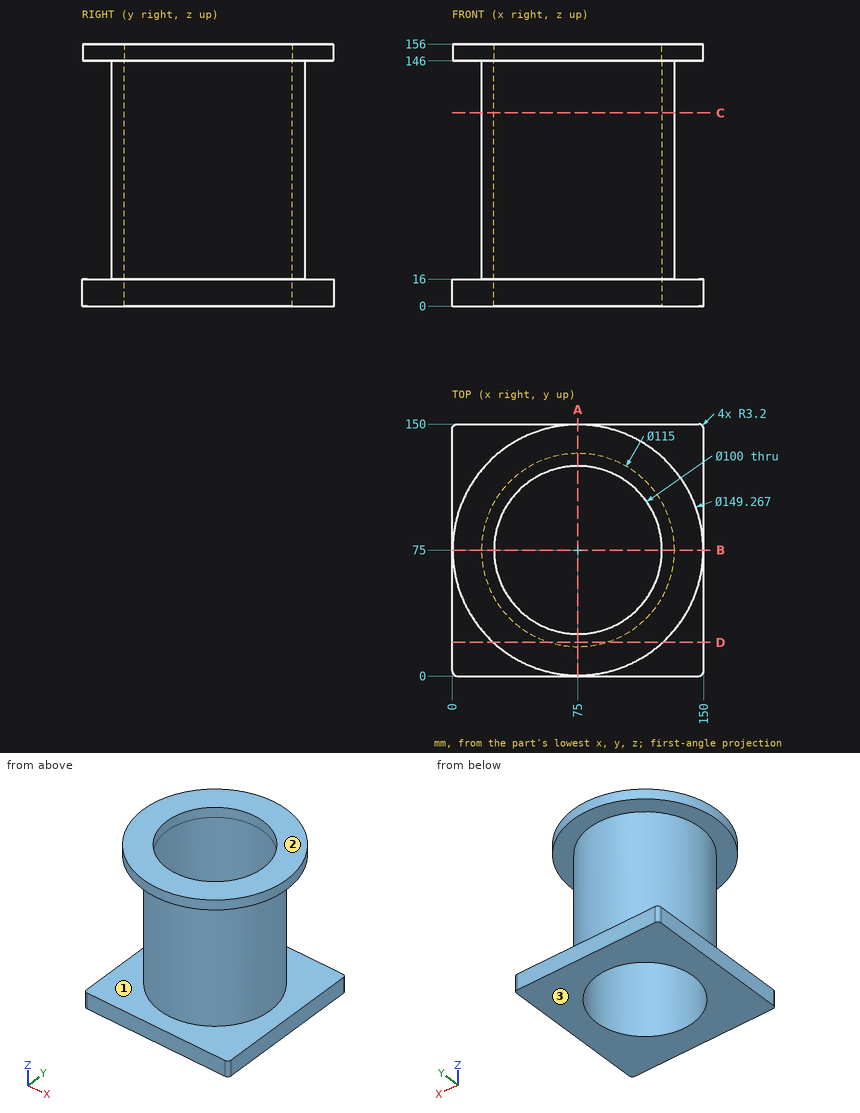
Here's the drawing with two shaded views (mm, measured from the low corner). I have some questions. Give positions to 0.01 mm unless a question says otherwise; leave off trailing zeros. Write each loop counter-clockwise with the first axis right and the second up, starting at its lowest first coordinate (ties: lowest second). Pieces come first, ordered by that corner, then holes. Notation, with made-up numbers: (-11, 16) -> (12, 16) arc R25 ccw to (12, 29) -> close; hole circle Ø4 at (37, -6.75). An arc over 180 degrees is marked (long way). Answer as a JSON object with one key per item and string values. Group by question number.
Item 1: We'd pull the mould along Z, two halves only. Please class the marked faces 1, 2 and 3: +Z half, -Z half, draft (parallel to the pull), parting line (faces both ways), or undercut.
Item 2: I'm going to push flat-ended pins straight in: P1, Ø8, axis at y = 127.5, z = 93.5, coming from the -X side; P2, Ø8, axis at y = 76, z = 34, coming from the -X side; P3, Ø4, axis at y = 89.5, z = 101.5, coming from the -X side (3 decimals). Where does each tip first touch, or does it pass through?
Item 3: Suppose I cut it at C-C (z = 115). Please give me the cut outline in (x, y).
Item 4: Please list where these lines run through material, in increasing order: line 1 (Z direction, x = 105.5, y = 21); line 2 (Y direction, x = 75, z = 105); line 3 (Y direction, x = 75, z = 152). Write a range as [from, to].
Item 5: Suppose I cut it at A-A (x = 75). Please give me the cut outline in (y, z).
Item 6: Suppose I cut it at D-D (y = 20). Please give me the cut outline in (x, z).
Findings:
{
 "1": {"face 1": "undercut", "face 2": "+Z half", "face 3": "-Z half"},
 "2": {"P1": "stops at x = 44.11", "P2": "stops at x = 17.5", "P3": "stops at x = 18.875"},
 "3": {"outline": "circle Ø115 at (75, 75); hole circle Ø100 at (75, 75)"},
 "4": {"line 1": "z = [0, 16], [146, 156]", "line 2": "y = [17.5, 25], [125, 132.5]", "line 3": "y = [0.37, 25], [125, 149.63]"},
 "5": {"outline": "(0, 0) -> (25, 0) -> (25, 156) -> (0.37, 156) -> (0.37, 146) -> (17.5, 146) -> (17.5, 16) -> (0, 16) -> close; (125, 0) -> (150, 0) -> (150, 16) -> (132.5, 16) -> (132.5, 146) -> (149.63, 146) -> (149.63, 156) -> (125, 156) -> close"},
 "6": {"outline": "(0, 0) -> (150, 0) -> (150, 16) -> (91.77, 16) -> (91.77, 146) -> (125.45, 146) -> (125.45, 156) -> (24.55, 156) -> (24.55, 146) -> (58.23, 146) -> (58.23, 16) -> (0, 16) -> close"}
}
